from build123d import *

# Parameters (mm, degrees)
BOSS_EXTRUDE1_DEPTH = 5.18
SKETCH3_R           = 9.5
BOSS_EXTRUDE2_DEPTH = 5
FILLET3_R           = 5
SKETCH4_R           = 6.9
CUT_EXTRUDE1_DEPTH  = 5
FILLET4_R           = 5


# Some blends are built 0.0001 mm under size
with BuildPart() as part:
    # Sketch1 → Boss-Extrude1 (new, symmetric)
    with BuildSketch(Plane(origin=(0, 0, 0), x_dir=(1, 0, 0), z_dir=(0, 1, 0))):
        Polygon((10.969655115, 0), (5.484827557, 9.5), (-5.484827557, 9.5), (-10.969655115, 0), (-5.484827557, -9.5), (5.484827557, -9.5), align=None)
    extrude(amount=BOSS_EXTRUDE1_DEPTH, both=True)

    # Sketch2 → Cut-Revolve1 (revolve, cut)
    with BuildSketch(Plane(origin=(0, 0, 0), x_dir=(0, 0, -1), z_dir=(1, 0, 0))):
        Polygon((-8.41, 5.18), (0, 5.18), (0, -5.18), (-7, -5.18), (-8.41, -4.36593612), (-7, -3.551872241), (-8.41, -2.737808361), (-7, -1.923744482), (-8.41, -1.109680602), (-7, -0.295616723), (-8.41, 0.518447157), (-7, 1.332511036), (-8.41, 2.146574916), (-7, 2.960638796), (-8.41, 3.774702675), (-7, 4.588766555), align=None)
    revolve(axis=Axis((0, 5.18, 0), (0, -1, 0)), mode=Mode.SUBTRACT)

    # Sketch3 → Boss-Extrude2 (add)
    with BuildSketch(Plane.XZ.offset(5.18)):
        with Locations(Location((0, 0, 0), (0, 0, 270))):
            Circle(SKETCH3_R)
    extrude(amount=BOSS_EXTRUDE2_DEPTH)

    # Fillet3
    fillet3_edges = [part.edges().sort_by_distance(p)[0] for p in [
        (0, -10.18, 9.5),
    ]]
    fillet(fillet3_edges, radius=FILLET3_R - 0.0001)  # a hair under: the kernel refuses the full size

    # Sketch4 → Cut-Extrude1 (cut)
    with BuildSketch(Plane.XZ.offset(10.18)):
        with Locations(Location((0, 0, 0), (0, 0, 270))):
            Circle(SKETCH4_R)
    extrude(amount=-CUT_EXTRUDE1_DEPTH, mode=Mode.SUBTRACT)

    # Fillet4
    # the kernel refuses this fillet: 5 mm, written as the material it takes off along each edge
    with BuildSketch(Plane(origin=(0, -5.18, 0), x_dir=(0, 0, -1), z_dir=(-1, 0, 0))) as fillet4_piece_1:
        with BuildLine():
            CenterArc((11.9, 0.994987437), FILLET4_R, 180, 11.478340955)
            Line((7, 0), (6.9, 0))
            Line((6.9, 0), (6.9, 0.994987437))
        make_face()
    revolve(axis=Axis((0, -5.18, 0), (0, -1, 0)), mode=Mode.SUBTRACT)


solid = part.part
Input: part model. Units: mm. Frame: model coordinates. A direction names the side the tool comes from. Give positions to 0.01 mm unless a question says otherwise; leave off trailing zeros. Write each loop counter-clockwise with the first axis right and the second up, starting at its lowest first coordinate (ties: lowest second). Pieces come first, ordered by that corner, then holes.
Q1. Section A-A, the plane y = 0. Output: boundary loops of the cut face in (x, z), plus the area to 3 significant figures.
Q2. Pull-direction query (X, two-part tool) for faces 1 (the face through (-8.2, 0.1, -4.8)), 2 (the face through (4.66, -7.89, 5.09)), 3 (the face through (5, -5.18, -9)); classes: pulls with the +X half, pulls with the -X half, needs draft (parallel to the pull), parting line crosses it, or undercut.
Q3. Set-up query: faces 4 (the face through (-5, -5.18, -9)), 5 (the face through (8.2, 0.1, 4.8)), 6 (the face through (0, 0, -9.5)), 7 (the face through (5, -5.18, 9)), 8 (the face through (-5, -5.18, 9)). Return all of +Z, -Z, +X, -X, +Y, -Y with unobstructed straight access to the full face (end or side cutting, diameter ignored); none if empty.
Q4. Section B-B, the plane z = -7.5. State how many separate pieces and enclosed holes the cut face has, plus the area to 3 significant figures.
Q5. Material intervals for probe 1 along Z at (x, y) = (-4.25, -2.25); probe 2 along X at (y, z) = (-7.75, -3.5); probe 3 along Z at (x, y) = (5.5, -2.5), sorted ascending.
Q6. First-contact query: P1, Ø3, axis at x = 1.5, z = -5.5, coming from the +Y side; P2, Ø1.4, axis at x = -9.5, z = 0, coming from the -Y side; P3, Ø2.5, axis at x = 4.5, z = 7.5, coming from the -Y side; P4, Ø11, axis at x = 0, z = 0, coming from the +Y side. Flat tips, straight axial feed; report the tip coordinate or a pass-through.
Filled in:
1. outline: (-10.97, 0) - (-5.48, -9.5) - (5.48, -9.5) - (10.97, 0) - (5.48, 9.5) - (-5.48, 9.5) - close; hole circle Ø15.02 at (0, 0)
1. area: 135 mm2
2. face 1: pulls with the -X half
2. face 2: undercut
2. face 3: needs draft
3. face 4: -Z, -X, -Y
3. face 5: +Z, +X, +Y, -Y
3. face 6: -Z, +X, -X, +Y, -Y
3. face 7: +Z, +X, -Y
3. face 8: +Z, -X, -Y
4. separate pieces: 1
4. enclosed holes: 6
4. area: 141 mm2
5. probe 1: z = -9.5 to -6.26, 6.26 to 9.5
5. probe 2: x = -8.06 to -5.95, 5.95 to 8.06
5. probe 3: z = -9.47 to -5.81, 5.81 to 9.47
6. P1: stops at y = 4.67
6. P2: stops at y = -7.73
6. P3: stops at y = -9.18
6. P4: passes through
